Print and shaded views of the part. All mm, measured from the part's lowest x, y and z. Round coordinates to 2 decimals unless told otherwise and drop trailing zeros. Loops run counter-clockwise (first coordinate to the right, second up) from the corner with the lowest first, then second, coordinate; pieces in that order, holes last. Notation, with made-up numbers: (-3, 62.25) -> (43, 62.25) arc R16 ccw to (43, 77.25) -> close; hole circle Ø8 at (77.25, -27). An arc over 180 degrees is marked (long way). Use a Markdown table: item, result.
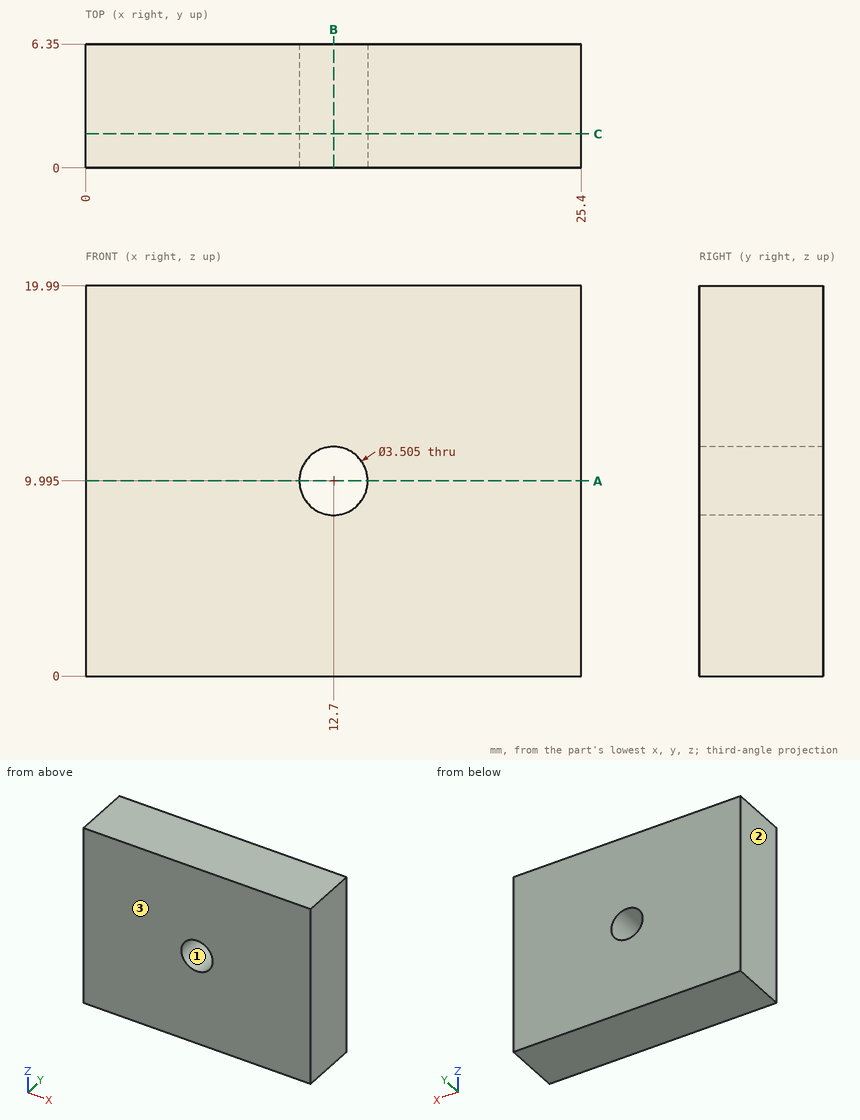
Q1. Band-saw the part on B-B, the plane x = 12.7. Give the cut face in (y, z).
Results list:
| item | result |
|---|---|
| outline | (0, 0) -> (6.35, 0) -> (6.35, 8.24) -> (0, 8.24) -> close; (0, 11.75) -> (6.35, 11.75) -> (6.35, 19.99) -> (0, 19.99) -> close |
Q2. Drill centre lines: L1, parallel to Z at x = 12.7, y = 2.25; L2, parallel to X at y = 1.5, z = 10.5; L3, parallel to X at y = 3.75, z = 8.75. Where is each one in solid material? Low to high. Write a range as from..to.
Results list:
| item | result |
|---|---|
| L1 | z = 0..8.24, 11.75..19.99 |
| L2 | x = 0..11.02, 14.38..25.4 |
| L3 | x = 0..11.47, 13.93..25.4 |
Q3. Band-saw the part on C-C, the plane y = 1.75. Give the cut face in (x, z) (1 decimal).
Results list:
| item | result |
|---|---|
| outline | (0, 0) -> (25.4, 0) -> (25.4, 20) -> (0, 20) -> close; hole circle Ø3.5 at (12.7, 10) |
Q4. Pull direction X, two halves, no side cores. Call the marked faces 1, 2 and 3: released by +X, released by -X, zero draft, split by the parting line, or undercut.
Results list:
| item | result |
|---|---|
| face 1 | undercut |
| face 2 | released by -X |
| face 3 | zero draft |
Q5. Band-saw the part on A-A, the plane z = 10. Give the cut face in (x, y).
Results list:
| item | result |
|---|---|
| outline | (0, 0) -> (10.95, 0) -> (10.95, 6.35) -> (0, 6.35) -> close; (14.45, 0) -> (25.4, 0) -> (25.4, 6.35) -> (14.45, 6.35) -> close |
